Build history of the part. All positions in model axes, mm. A direction names the side the tool comes from. Coordinates: 2 decimals unless noted, no trailing zeros. Write each loop counter-clockwise with the first axis right and the second up, starting at its lowest first coordinate (ties: lowest second). Pieces come first, ordered by that corner, then holes. Notation, with made-up numbers: M 55,74 L 83,74 A11 cw 83,89 Z; hole C 25,66.25 d8. An arc over 180 degrees is marked long. Use CSV: the item, a comma, the result in double quotes. Start each with the question number.
```python
from build123d import *

# Parameters (mm, degrees)
F1_DEPTH = 20
F3_DEPTH = 20
F5_DEPTH = 20


with BuildPart() as f1:
    # F0 (on Front) → F1 (new body)
    with BuildSketch(Plane.XZ):
        Polygon((-24.709278, 32.928156), (-54.709278, 32.928156), (-54.709278, -32.071844), (35.290722, -32.071844), (35.290722, 32.928156), (5.290722, 32.928156), (5.290722, 7.385719), (-24.709278, 7.385719), align=None)
    extrude(amount=F1_DEPTH)

    # F2 (on face) → F3 (join)
    with BuildSketch(Plane.XZ.offset(20)):
        Polygon((-54.709278, 32.928156), (-54.709278, -32.071844), (-24.709278, -32.071844), align=None)
    extrude(amount=F3_DEPTH)

    # F4 (on face) → F5 (join)
    with BuildSketch(Plane.XZ.offset(20)):
        Polygon((5.290722, -32.071844), (35.290722, -32.071844), (35.290722, 32.928156), align=None)
    extrude(amount=F5_DEPTH)


solid = f1.part
```
1. Slice it at D-D (x = 29). List the corners of the cut face in (y, z), and give its area (3 significant figures).
2. Slice it at C-C (y = -11). List the corners of the cut face in (x, z), and give its area (3 significant figures).
3. Pull direction X, two halves, no side cores. Call faces 4 (the flat face through (-9, -10, 7.386)), 5 (the flat face through (-10.3, -19.7, -32.072)), 6 (the flat face through (35.291, -20, 0)): pulls with the +X half, pulls with the -X half, needs draft (parallel to the pull), parting line crosses it, or undercut.
4. Drill centre lines: line 1 along X through (y, z) = (-9, 19.5); line 2 along Y through (x, z) = (15, -10); line 3 along X through (y, z) = (-21.5, -23). Where is each one in solid material? Low to high. Write a range as from..to.
5. 3-axis set-ups, long thin cutter, end or side, ignore diameter. For faces 1 (the flat face through (20.5, -29.86, 0.88)), 2 (the flat face through (-54.709, -20, 1)), 3 (the flat face through (5.291, -10, 20)): which of +Z, -Z, +X, -X, +Y, -Y reach the whole face in a straight line?
6. Slice it at B-B (z = 27.5). List the corners of the cut face in (x, y).
7. Flat gauge pins, fed straight in: pin 1 (22 mm diameter, centred on x = -5.5, y = -7.5, fed in from +Z); pin 2 (10 mm diameter, centred on x = -21, y = -23.5, fed in from +Z); pin 3 (8 mm diameter, centred on x = -10, z = 10.5, fed in from -Y). Where does each tip first touch, or does it go through?
8. Slice it at A-A (y = -30). List the corners of the cut face in (x, z).
Established:
1,outline,"M -40,-32.07 L 0,-32.07 L 0,32.93 L -20,32.93 L -20,19.3 L -40,19.3 Z"
1,area,"2,330 mm2"
2,outline,"M -54.71,-32.07 L 35.29,-32.07 L 35.29,32.93 L 5.29,32.93 L 5.29,7.39 L -24.71,7.39 L -24.71,32.93 L -54.71,32.93 Z"
2,area,"5,080 mm2"
3,face 4,"undercut"
3,face 5,"needs draft"
3,face 6,"pulls with the +X half"
4,line 1,"x = -54.71..-24.71, 5.29..35.29"
4,line 2,"y = -20..0"
4,line 3,"x = -54.71..-28.9, 9.48..35.29"
5,face 1,"+Z, -Y"
5,face 2,"+Z, -Z, -X, +Y, -Y"
5,face 3,"+Z, +Y, -Y"
6,outline,"M -54.71,-40 L -52.2,-40 L -52.2,-20 L -24.71,-20 L -24.71,0 L -54.71,0 Z; M 5.29,-20 L 32.79,-20 L 32.79,-40 L 35.29,-40 L 35.29,0 L 5.29,0 Z"
7,pin 1,"stops at z = 32.93"
7,pin 2,"stops at z = 7.39"
7,pin 3,"stops at y = -20"
8,outline,"M -54.71,-32.07 L -24.71,-32.07 L -54.71,32.93 Z; M 5.29,-32.07 L 35.29,-32.07 L 35.29,32.93 Z"
